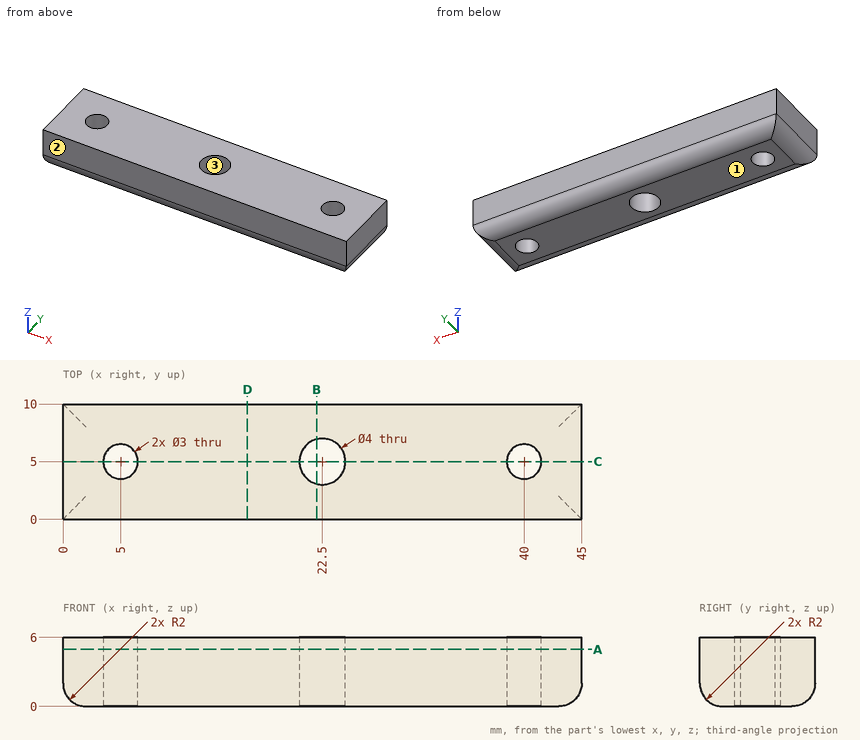
Answer from the drawing. Dimensions are ordinates in mm from the lowest x, y and z of the part. Round coordinates to 2 decimals unless told otherwise and drop trailing zeros. Write each loop counter-clockwise with the first axis right and the second up, starting at its lowest first coordinate (ties: lowest second). Pieces come first, ordered by that corner, then holes. Notation, with made-up numbers: (-27.5, -6) -> (19.5, -6) arc R23 cw to (19.5, 23) -> close; hole circle Ø10 at (76.5, 77.5). An arc over 180 degrees is marked (long way). Write each question's results on one line, items separated by ' | '.
1) Consider line 1 along Y through (x, z) = (22.5, 3); line 2 along Y through (x, z) = (40, 2.7); line 3 along X through (y, z) = (5.75, 1.65). Determine where each line is inside the solid, lowest interval first. Write a range as [from, to].
Findings:
line 1: y = [0, 3], [7, 10] | line 2: y = [0, 3.5], [6.5, 10] | line 3: x = [0.03, 3.7], [6.3, 20.65], [24.35, 38.7], [41.3, 44.97]
2) The part is cut by section B-B (x = 22). Write down the section's boundary in (y, z).
Findings:
outline: (0, 2) arc R2 ccw to (2, 0) -> (3.06, 0) -> (3.06, 6) -> (0, 6) -> close; (6.94, 0) -> (8, 0) arc R2 ccw to (10, 2) -> (10, 6) -> (6.94, 6) -> close
3) The part is cut by section C-C (y = 5). Write down the section's boundary in (x, z).
Findings:
outline: (0, 2) arc R2 ccw to (2, 0) -> (3.5, 0) -> (3.5, 6) -> (0, 6) -> close; (6.5, 0) -> (20.5, 0) -> (20.5, 6) -> (6.5, 6) -> close; (24.5, 0) -> (38.5, 0) -> (38.5, 6) -> (24.5, 6) -> close; (41.5, 0) -> (43, 0) arc R2 ccw to (45, 2) -> (45, 6) -> (41.5, 6) -> close
4) The part is cut by section D-D (x = 16). Write down the section's boundary in (y, z), and give its area (3 significant figures).
Findings:
outline: (0, 2) arc R2 ccw to (2, 0) -> (8, 0) arc R2 ccw to (10, 2) -> (10, 6) -> (0, 6) -> close | area: 58.3 mm²
5) The part is cut by section A-A (z = 4.95). Write down the section's boundary in (x, y), and give its area (3 significant figures).
Findings:
outline: (0, 0) -> (45, 0) -> (45, 10) -> (0, 10) -> close; hole circle Ø3 at (5, 5); hole circle Ø4 at (22.5, 5); hole circle Ø3 at (40, 5) | area: 423 mm²
6) For a pull along Y with two mould halves and no side action, classify the marked faces 1, 2 and 3 as +Y half, -Y half, draft (parallel to the pull), parting line (faces both ways), or undercut.
Findings:
face 1: draft | face 2: -Y half | face 3: undercut
